The listing builds one solid part. Answer for the finished solid, in the listing's coordinates (mm). Give positions to 0.01 mm unless a question says otherwise; leave off trailing zeros. Order: outer loops, then holes, each group sorted by start corner. A loop starts at its lowest first (then second) coordinate and runs counter-clockwise, first axis right, second up. Notation, with made-up numbers: M 42,42 L 81,42 A26 cw 81,76 Z; hole C 79,19.5 d6. An arc over 180 degrees is marked long. Answer as a JSON object with one key per item and string values. Group by question number.
Autodesk Inventor part; units mm, degrees
ref_plane "YZ Plane" through (0, 0, 0) normal (1, 0, 0) x (0, 1, 0)
ref_plane "XZ Plane" through (0, 0, 0) normal (0, 1, 0) x (-1, 0, 0)
ref_plane "XY Plane" through (0, 0, 0) normal (0, 0, 1) x (1, 0, 0)
sketch "Sketch1" plane through (0, 0, 0) normal (0, 0, 1) x (1, 0, 0)
  line L0 (-39.5223, 4.2825) -> (17.4753, 4.2825)
  line L1 (17.4753, 4.2825) -> (17.4753, -52.7151)
  line L2 (17.4753, -52.7151) -> (-39.5223, -52.7151)
  line L3 (-39.5223, -52.7151) -> (-39.5223, 4.2825)
  circle A0 centre (-34.5937, -47.7865) radius 2.5527
  circle A1 centre (12.5467, -47.7865) radius 2.5527
  circle A2 centre (-34.5937, -0.6461) radius 2.5527
  circle A3 centre (12.5467, -0.6461) radius 2.5527
  line L4 (-68.1735, 24.6219) -> (-42.7735, 24.6219)
  line L5 (-42.7735, 24.6219) -> (-42.7735, -38.8781)
  line L6 (-42.7735, -38.8781) -> (-68.1735, -38.8781)
  line L7 (-68.1735, -38.8781) -> (-68.1735, 24.6219)
  circle A4 centre (-55.4735, 18.2719) radius 2.6543
  circle A5 centre (-55.4735, -32.5281) radius 2.6543
  circle A6 centre (-55.4735, -7.1281) radius 2.6543
  line L8 (-68.1735, -7.1281) -> (-42.7735, -7.1281)
  circle A7 centre (-55.4735, 46.8469) radius 8.6868
  line L9 (-42.7735, 24.6219) -> (17.4753, 4.2825)
  line L10 (-68.1735, -38.8781) -> (-39.5223, -52.7151)
  circle A8 centre (-11.0235, -24.2163) radius 3.81
  point P0 (0, 0)
  dimension "d0" = 56.9976
  dimension "d1" = 56.9976
  dimension "d3" = 5.1054
  dimension "d4" = 5.1054
  dimension "d5" = 5.1054
  dimension "d7" = 5.1054
  dimension "d15" = 28.4988
  dimension "d16" = 28.4988
  dimension "d17" = 63.5
  dimension "d18" = 25.4
  dimension "d19" = 25.4
  dimension "d20" = 0
  dimension "d21" = 5.3086
  dimension "d22" = 5.3086
  dimension "d23" = 5.3086
  dimension "d24" = 28.575
  dimension "d26" = 12.7
  dimension "d28" = 0
  dimension "d29" = 0
  dimension "d30" = 12.7
  dimension "d33" = 83.82
  dimension "d34" = 44.45
  dimension "d37" = 7.62
  dimension "d39" = 66.6666
  dimension "d40" = 66.6666
  dimension "d41" = 33.3333
  dimension "d42" = 33.3333
extrude "Extrusion1" add sketch "Sketch1" along normal blind 3.175 contours L3 L10 L6 L5 L9 L0 | L0 L1 L2 L3 | L5 L8 A6 L7 L4 | L7 L8 A6 L5 L6
fillet "Fillet1" radius 6.35 6 edges at (-42.7735, 24.6219, 1.5875) (-68.1735, 24.6219, 1.5875) (17.4753, 4.2825, 1.5875) (17.4753, -52.7151, 1.5875) (-39.5223, -52.7151, 1.5875) (-68.1735, -38.8781, 1.5875)
equation "\"d4\" = d3"
equation "\"d19\" = d18"
equation "\"d22\" = d21"
equation "\"d23\" = d21"
equation "\"d40\" = d39"
equation "\"d41\" = 0.5 * d39"
properties part number "Diff Motor Bracket"
Item 1: Consider probe 1 along Y at (x, z) = (12, 1.9); probe 2 along X at (y, z) = (-27, 0.35); probe 3 along X at (y, z) = (-23, 0.65). Determine where each line is inside the solid, lowest interval first. Write a range as from..to.
Item 2: A flat-ended cylindrical pin translates along its axis: P1, Ø1, axis at x = -39, z = 0.5, coming from the -Y side. Find the tip coordinate at first contact, or state that the pin passes through.
Item 3: Section C-C (x = -10.5) is taken. Determine the outline of the cut face in (y, z) (3 decimals), and give its area (3 significant figures).
Item 4: Section D-D (z = 0.8) is taken. Count the separate pieces of the cut face and the enclosed holes in it, and give its area (3 significant figures).
Item 5: Section B-B (y = -2) is taken. Determine the outline of the cut face in (x, z) (1 decimal), and give its area (3 significant figures).
Item 6: Determine the mould class of faces 1 (the cylindrical face through (-34.926, -50.317, 1.565)), 2 (the flat face through (-68.174, -9, 2)), 3 (the cylindrical face through (15.57, -50.9, 1.61)) for opening direction X: released by +X, released by -X, zero draft, split by the parting line, or undercut.
Item 7: Section A-A (x = -57) is taken. Determine the outline of the cut face in (y, z) (3 decimals).
Values found:
{
 "1": {"probe 1": "y = -52.65..-50.28, -45.29..-3.14, 1.85..6.13", "probe 2": "x = -68.17..-13.62, -8.42..17.48", "probe 3": "x = -68.17..-14.63, -7.41..17.48"},
 "2": {"P1": "stops at y = -52.7"},
 "3": {"outline": "M -52.715,0 L -27.99,0 L -27.99,3.175 L -52.715,3.175 Z; M -20.442,0 L 13.727,0 L 13.727,3.175 L -20.442,3.175 Z", "area": "187 mm^2"},
 "4": {"separate pieces": "1", "enclosed holes": "8", "area": "5,590 mm^2"},
 "5": {"outline": "M -68.2,0 L -36.8,0 L -36.8,3.2 L -68.2,3.2 Z; M -32.4,0 L 10.4,0 L 10.4,3.2 L -32.4,3.2 Z; M 14.7,0 L 17.5,0 L 17.5,3.2 L 14.7,3.2 Z", "area": "244 mm^2"},
 "6": {"face 1": "undercut", "face 2": "released by -X", "face 3": "released by +X"},
 "7": {"outline": "M -44.274,0 L -34.7,0 L -34.7,3.175 L -44.274,3.175 Z; M -30.357,0 L -9.3,0 L -9.3,3.175 L -30.357,3.175 Z; M -4.957,0 L 16.1,0 L 16.1,3.175 L -4.957,3.175 Z; M 20.443,0 L 24.622,0 L 24.622,3.175 L 20.443,3.175 Z"}
}
